Geometry check sheet. Reference: the model listing, model coordinates, mm. Face numbers are marked on the shaded views. A direction names the side the tool comes from. Round coordinates to 2 decimals unless told otherwise and drop trailing zeros. Loops run counter-clockwise (first coordinate to the right, second up) from the corner with the lowest first, then second, coordinate; pieces in that order, holes last. Notation, with made-up numbers: (54, -12.75) - (89, -12.75) arc R16 ccw to (89, 9.25) - close; hole circle Ø11 at (23.25, 32). An arc over 180 degrees is marked (long way). Write item = value, one per line.
```python
from build123d import *

# Parameters (mm, degrees)
F0_R     = 20
F1_DEPTH = 10
F2_R     = 12
F3_DEPTH = 30
F4_R     = 6
F5_DEPTH = 40.001
F7_DEPTH = 25
F9_D     = 6


with BuildPart() as f1:
    # F0 (on Front) → F1 (new body)
    with BuildSketch(Plane.XZ):
        Circle(F0_R)
    extrude(amount=F1_DEPTH)

    # F2 (on face) → F3 (join)
    with BuildSketch(Plane.XZ.offset(10)):
        Circle(F2_R)
    extrude(amount=F3_DEPTH)

    # F4 (on face) → F5 (cut, through all)
    with BuildSketch(Plane.XZ.offset(40)):
        Circle(F4_R)
    extrude(amount=-F5_DEPTH, mode=Mode.SUBTRACT)

    # F6 (on face) → F7 (cut)
    with BuildSketch(Plane(origin=(0, 0, 0), x_dir=(-1, 0, 0), z_dir=(0, 1, 0))):
        with BuildLine():
            Line((-15, -13.228757), (-15, 0))
            Line((-15, 0), (-15, 13.228757))
            ThreePointArc((-15, 13.228757), (-20, 0), (-15, -13.228757))
        make_face()
        with BuildLine():
            ThreePointArc((20, 0), (18.708287, 7.071068), (15, 13.228757))
            Line((15, 13.228757), (15, 0))
            Line((15, 0), (15, -13.228757))
            ThreePointArc((15, -13.228757), (18.708287, -7.071068), (20, 0))
        make_face()
    extrude(amount=-F7_DEPTH, mode=Mode.SUBTRACT)

    # F9 (through all)
    with Locations(Plane(origin=(0, 0, 0), x_dir=(-1, 0, 0), z_dir=(0, 1, 0))):
        with Locations((-11.313708, 11.313708), (0, 16), (11.313708, 11.313708), (-11.313708, -11.313708), (0, -16), (11.313708, -11.313708)):
            Hole(F9_D / 2)


solid = f1.part
```
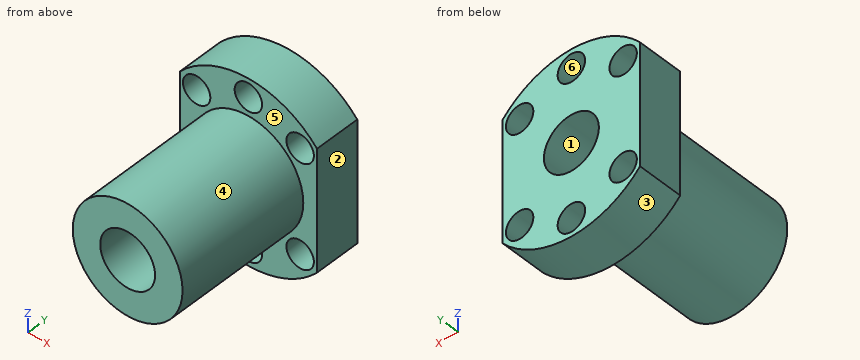
(1) Mould release check, pull along Z, two halves, no side actions. Record for the marked faces 1, 2, 3 and 4: pulls with the +Z half, pulls with the -Z half, needs draft (parallel to the pull), parting line crosses it, or undercut.
Answers follow:
face_1 = undercut
face_2 = needs draft
face_3 = pulls with the -Z half
face_4 = parting line crosses it
(2) Section check C-C (x = 10). Enter the section's corners in (y, z), then the cut area to 3 significant figures.
Answers follow:
outline = (-40, -6.63) - (-10, -6.63) - (-10, -8.62) - (0, -8.62) - (0, 8.62) - (-10, 8.62) - (-10, 6.63) - (-40, 6.63) - close; (-10, -17.32) - (0, -17.32) - (0, -14.01) - (-10, -14.01) - close; (-10, 14.01) - (0, 14.01) - (0, 17.32) - (-10, 17.32) - close
area = 637 mm²
(3) Scan lines: L1, parallel to Z at x = 0, y = -1.75; L2, parallel to X at y = -2, z = 13.5; L3, parallel to X at y = -4.5, z = -9. Record each from-to range of solid material in increasing order. Write a range as [from, to].
Answers follow:
L1 = [-20, -19], [-13, -6], [6, 13], [19, 20]
L2 = [-14.76, -13.37], [-9.26, -1.66], [1.66, 9.26], [13.37, 14.76]
L3 = [-15, -13.22], [-9.4, 9.4], [13.22, 15]
(4) Gauge pin test, flat ends, axial feed: pin 1 (12 mm diameter, centred on x = 0.5, y = -35.5, fed in from +Z); pin 2 (4 mm diameter, centred on x = 1.5, y = -8.5, fed in from -Z); pin 3 (10 mm diameter, centred on x = 6, y = -25.5, fed in from -Z). Record the tip position at first contact, or that the pin passes through.
Answers follow:
pin_1 = 12
pin_2 = -20
pin_3 = -11.96
(5) Section check D-D (z = -10). Enter the section's corners in (x, y), then the cut area to 3 significant figures.
Answers follow:
outline = (-15, -10) - (-14.01, -10) - (-14.01, 0) - (-15, 0) - close; (-8.62, -10) - (-6.63, -10) - (-6.63, -40) - (6.63, -40) - (6.63, -10) - (8.62, -10) - (8.62, 0) - (-8.62, 0) - close; (14.01, -10) - (15, -10) - (15, 0) - (14.01, 0) - close
area = 590 mm²
(6) Section check A-A (z = -16). Enter the section's corners in (x, y).
Answers follow:
outline = (-12, -10) - (-3, -10) - (-3, 0) - (-12, 0) - close; (3, -10) - (12, -10) - (12, 0) - (3, 0) - close
(7) Section check B-B (x = -2). Enter the section's corners in (y, z), then the cut area to 3 significant figures.
Answers follow:
outline = (-40, -11.83) - (-10, -11.83) - (-10, -13.76) - (0, -13.76) - (0, -5.66) - (-40, -5.66) - close; (-40, 5.66) - (0, 5.66) - (0, 13.76) - (-10, 13.76) - (-10, 11.83) - (-40, 11.83) - close; (-10, -19.9) - (0, -19.9) - (0, -18.24) - (-10, -18.24) - close; (-10, 18.24) - (0, 18.24) - (0, 19.9) - (-10, 19.9) - close
area = 566 mm²
(8) Set-up check for the marked faces 5 and 6: record each of +Z, -Z, +X, -X, +Y, -Y from which the full face is reachable in a straight line by a thin tool's end or side.
Answers follow:
face_5 = -Y
face_6 = +Y, -Y
